For this review, take the finished solid that the model builds, in its own axes (mm). Coordinates: 2 decimals unless noted, no trailing zeros. Loops run counter-clockwise (first coordinate to the right, second up) from the corner with the lowest first, then second, coordinate; pieces in that order, holes last. Notation, with made-up numbers: (-10, 89) -> (-2, 89) arc R21 cw to (-2, 97) -> close; hole circle Ø11 at (32, 46). An arc over 180 degrees is marked (long way). Answer in a Markdown table with one row per item.
from build123d import *

# Parameters (mm, degrees)
SKETCH_1_W          = 10
SKETCH_1_H          = 10
EXTRUDE_1_DEPTH     = 3
SKETCH_2_R          = 1.25
CUT_EXTRUDE_1_DEPTH = 7
SKETCH_3_R          = 1.25
CUT_EXTRUDE_2_DEPTH = 11
SKETCH_4_R          = 1.25
CUT_EXTRUDE_3_DEPTH = 11


with BuildPart() as part:
    # 草圖1 → 填料-伸長1 (new body, symmetric)
    with BuildSketch(Plane(origin=(0, 0, 0), x_dir=(1, 0, 0), z_dir=(0, 1, 0))):
        Rectangle(SKETCH_1_W, SKETCH_1_H)
    extrude(amount=EXTRUDE_1_DEPTH, both=True)

    # 草圖2 → 除料-伸長1 (cut, through all)
    with BuildSketch(Plane(origin=(0, 3, 0), x_dir=(1, 0, 0), z_dir=(0, 1, 0))):
        Circle(SKETCH_2_R)
    extrude(amount=-CUT_EXTRUDE_1_DEPTH, mode=Mode.SUBTRACT)

    # 草圖3 → 除料-伸長2 (cut, through all)
    with BuildSketch(Plane.XY.offset(5)):
        Circle(SKETCH_3_R)
    extrude(amount=-CUT_EXTRUDE_2_DEPTH, mode=Mode.SUBTRACT)

    # 草圖4 → 除料-伸長3 (cut, through all)
    with BuildSketch(Plane(origin=(5, 0, 0), x_dir=(0, 0, -1), z_dir=(1, 0, 0))):
        Circle(SKETCH_4_R)
    extrude(amount=-CUT_EXTRUDE_3_DEPTH, mode=Mode.SUBTRACT)


solid = part.part
Item 1: Insertion check: pin 1 (3 mm diameter, centred on x = 0, z = 0, fed in from +Y). The pin has a flat end and moves straight along its axis. Give the tip position at first contact, or say it passes through.
Worked answers:
| item | result |
|---|---|
| pin 1 | y = 3 |
Item 2: Take a section at B-B, the plane z = 0.75. State the section outline as (x, y) points, and give its area (3 significant figures).
Worked answers:
| item | result |
|---|---|
| outline | (-5, -3) -> (-1, -3) -> (-1, -1) -> (-5, -1) -> close; (-5, 1) -> (-1, 1) -> (-1, 3) -> (-5, 3) -> close; (1, -3) -> (5, -3) -> (5, -1) -> (1, -1) -> close; (1, 1) -> (5, 1) -> (5, 3) -> (1, 3) -> close |
| area | 32.0 mm² |
Item 3: Take a section at D-D, the plane x = -2.5. State the section outline as (y, z) points, and give its area (3 significant figures).
Worked answers:
| item | result |
|---|---|
| outline | (-3, -5) -> (3, -5) -> (3, 5) -> (-3, 5) -> close; hole circle Ø2.5 at (0, 0) |
| area | 55.1 mm² |
Item 4: The part is to be moulded in two halves that separate along Y. For faces 1 (the flat face through (-5, 1, 1)), 2 (the cylindrical face through (2.97, 0.05, 1.25)), 3 (the flat face through (-1, -3, 1)), say which applies: +Y half, -Y half, draft (parallel to the pull), parting line (faces both ways), or undercut.
Worked answers:
| item | result |
|---|---|
| face 1 | draft |
| face 2 | undercut |
| face 3 | -Y half |
Item 5: For L1, parallel to X at y = 0, z = -1.9; L2, parallel to Y at x = 3.3, z = 0, list the stretches that pass through material, from the lowest coordinate up.
Worked answers:
| item | result |
|---|---|
| L1 | -5 to -1.25, 1.25 to 5 |
| L2 | -3 to -1.25, 1.25 to 3 |
Item 6: Take a section at A-A, the plane x = 0. State the section outline as (y, z) points.
Worked answers:
| item | result |
|---|---|
| outline | (-3, -5) -> (-1.25, -5) -> (-1.25, -1.25) -> (-3, -1.25) -> close; (-3, 1.25) -> (-1.25, 1.25) -> (-1.25, 5) -> (-3, 5) -> close; (1.25, -5) -> (3, -5) -> (3, -1.25) -> (1.25, -1.25) -> close; (1.25, 1.25) -> (3, 1.25) -> (3, 5) -> (1.25, 5) -> close |
Item 7: Take a section at C-C, the plane z = 4. State the section outline as (x, y) points.
Worked answers:
| item | result |
|---|---|
| outline | (-5, -3) -> (5, -3) -> (5, 3) -> (-5, 3) -> close; hole circle Ø2.5 at (0, 0) |
